from build123d import *

# Parameters (mm, degrees)
SKETCH_1_R          = 41.5
SKETCH_1_R_2        = 2
SKETCH_1_R_3        = 14
EXTRUDE_1_DEPTH     = 2
CUT_EXTRUDE_3_DEPTH = 2
FILLET_1_R          = 1
SKETCH_5_R          = 1.65
CUT_EXTRUDE_4_DEPTH = 10
SKETCH_6_R          = 2.5
CUT_EXTRUDE_5_DEPTH = 10


with BuildPart() as part:
    # 草图1 → 凸台-拉伸1 (new body)
    with BuildSketch(Plane.XY):
        Circle(SKETCH_1_R)
        with Locations((0, -37)):
            Circle(SKETCH_1_R_2, mode=Mode.SUBTRACT)
        with Locations((-37, 0)):
            Circle(SKETCH_1_R_2, mode=Mode.SUBTRACT)
        with Locations((0, 37)):
            Circle(SKETCH_1_R_2, mode=Mode.SUBTRACT)
        with Locations((37, 0)):
            Circle(SKETCH_1_R_2, mode=Mode.SUBTRACT)
        Circle(SKETCH_1_R_3, mode=Mode.SUBTRACT)
    extrude(amount=EXTRUDE_1_DEPTH)

    # 草图4 → 切除-拉伸3 (cut)
    with BuildSketch(Plane.XY.offset(2)):
        with BuildLine():
            ThreePointArc((-10.565456544, 22.657694676), (-17.67766953, 17.67766953), (-22.657694676, 10.565456544))
            Line((-22.657694676, 10.565456544), (-27.189233611, 12.678547852))
            ThreePointArc((-27.189233611, 12.678547852), (-21.213203436, 21.213203436), (-12.678547852, 27.189233611))
            Line((-12.678547852, 27.189233611), (-10.565456544, 22.657694676))
        make_face()
        with BuildLine():
            Line((22.657694676, 10.565456544), (27.189233611, 12.678547852))
            ThreePointArc((27.189233611, 12.678547852), (21.213203436, 21.213203436), (12.678547852, 27.189233611))
            Line((12.678547852, 27.189233611), (10.565456544, 22.657694676))
            ThreePointArc((10.565456544, 22.657694676), (17.67766953, 17.67766953), (22.657694676, 10.565456544))
        make_face()
        with BuildLine():
            ThreePointArc((-22.657694676, -10.565456544), (-17.67766953, -17.67766953), (-10.565456544, -22.657694676))
            Line((-10.565456544, -22.657694676), (-12.678547852, -27.189233611))
            ThreePointArc((-12.678547852, -27.189233611), (-21.213203436, -21.213203436), (-27.189233611, -12.678547852))
            Line((-27.189233611, -12.678547852), (-22.657694676, -10.565456544))
        make_face()
        with BuildLine():
            ThreePointArc((10.565456544, -22.657694676), (17.67766953, -17.67766953), (22.657694676, -10.565456544))
            Line((22.657694676, -10.565456544), (27.189233611, -12.678547852))
            ThreePointArc((27.189233611, -12.678547852), (21.213203436, -21.213203436), (12.678547852, -27.189233611))
            Line((12.678547852, -27.189233611), (10.565456544, -22.657694676))
        make_face()
    extrude(amount=-CUT_EXTRUDE_3_DEPTH, mode=Mode.SUBTRACT)

    # 圆角1
    fillet_1_edges = [part.edges().sort_by_distance(p)[0] for p in [
        (27.189233611, 12.678547852, 1),
        (22.657694676, 10.565456544, 1),
        (10.565456544, 22.657694676, 1),
        (12.678547852, 27.189233611, 1),
        (-22.657694676, -10.565456544, 1),
        (-10.565456544, -22.657694676, 1),
        (-12.678547852, -27.189233611, 1),
        (-27.189233611, -12.678547852, 1),
        (10.565456544, -22.657694676, 1),
        (22.657694676, -10.565456544, 1),
        (27.189233611, -12.678547852, 1),
        (12.678547852, -27.189233611, 1),
        (-10.565456544, 22.657694676, 1),
        (-22.657694676, 10.565456544, 1),
        (-27.189233611, 12.678547852, 1),
        (-12.678547852, 27.189233611, 1),
    ]]
    fillet(fillet_1_edges, radius=FILLET_1_R)

    # 草图5 → 切除-拉伸4 (cut)
    with BuildSketch(Plane.XY.offset(2)):
        with Locations((-17.320508076, 10)):
            Circle(SKETCH_5_R)
        with Locations((17.320508076, 10)):
            Circle(SKETCH_5_R)
        with Locations((0, -20)):
            Circle(SKETCH_5_R)
    extrude(amount=-CUT_EXTRUDE_4_DEPTH, mode=Mode.SUBTRACT)

    # 草图6 → 切除-拉伸5 (cut)
    with BuildSketch(Plane.XY.offset(2)):
        with Locations((-17.320508076, -10)):
            Circle(SKETCH_6_R)
    extrude(amount=-CUT_EXTRUDE_5_DEPTH, mode=Mode.SUBTRACT)


solid = part.part
The listing builds one solid part. Answer for the finished solid, in the listing's coordinates (mm). Give positions to 0.01 mm unless a question says otherwise; leave off trailing zeros. Loops run counter-clockwise (first coordinate to the right, second up) from the corner with the lowest first, then second, coordinate; pieces in that order, holes last. Notation, with made-up numbers: (-38, -10.5) - (8, -10.5) arc R7 ccw to (8, -5.5) - close; hole circle Ø11 at (38.25, 86). An arc over 180 degrees is marked (long way). Write each question's results on one line, items separated by ' | '.
1. Consider probe 1 along Y at (x, z) = (0, 1.3); probe 2 along Y at (x, z) = (23, 0.5); probe 3 along X at (y, z) = (13, 1.05). Determine where each line is inside the solid, lowest interval first. Write a range as from..to.
Resolved:
probe 1: y = -41.5..-39, -35..-21.65, -18.35..-14, 14..35, 39..41.5 | probe 2: y = -34.54..-19.26, -10.89..10.89, 19.26..34.54 | probe 3: x = -39.41..-26.83, -21.35..-5.2, 5.2..21.35, 26.83..39.41
2. For a pull along X with two mould halves and no side action, classify faces 1 (the face through (-24.926, -11.623, 1.014)), 2 (the face through (-1, -18, 2)) as +X half, -X half, draft (parallel to the pull), parting line (faces both ways), or undercut.
Resolved:
face 1: undercut | face 2: draft
3. Find section A-A, the plane y = 0. Write down the section's boundary in (x, z), then the cut area to 3 significant figures.
Resolved:
outline: (-41.5, 0) - (-39, 0) - (-39, 2) - (-41.5, 2) - close; (-35, 0) - (-14, 0) - (-14, 2) - (-35, 2) - close; (14, 0) - (35, 0) - (35, 2) - (14, 2) - close; (39, 0) - (41.5, 0) - (41.5, 2) - (39, 2) - close | area: 94.0 mm^2
4. Find section C-C, the plane y = -37. Write down the section's boundary in (x, z).
Resolved:
outline: (-18.79, 0) - (-2, 0) - (-2, 2) - (-18.79, 2) - close; (2, 0) - (18.79, 0) - (18.79, 2) - (2, 2) - close
5. Find section B-B, the plane x = 0. Write down the section's boundary in (y, z), then the cut area to 3 significant figures.
Resolved:
outline: (-41.5, 0) - (-39, 0) - (-39, 2) - (-41.5, 2) - close; (-35, 0) - (-21.65, 0) - (-21.65, 2) - (-35, 2) - close; (-18.35, 0) - (-14, 0) - (-14, 2) - (-18.35, 2) - close; (14, 0) - (35, 0) - (35, 2) - (14, 2) - close; (39, 0) - (41.5, 0) - (41.5, 2) - (39, 2) - close | area: 87.4 mm^2
